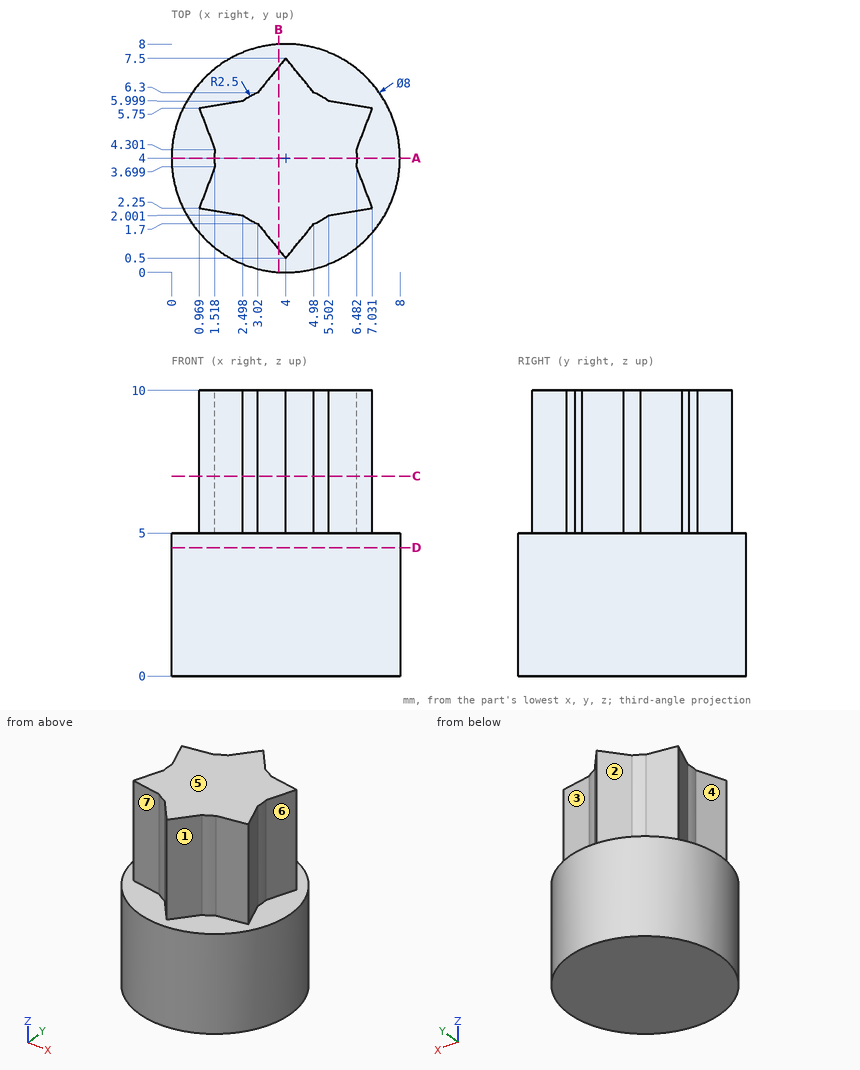
Verification items for this drawing (mm, ordinates from the low corner). A direction names the side the tool comes from. Coordinates: 2 decimals unless noted, no trailing zeros. Order: outer loops, then holes, each group sorted by start corner. A loop starts at its lowest first (then second) coordinate and runs counter-clockwise, first axis right, second up. Notation, with made-up numbers: (7.5, 23) - (59.5, 23) arc R8 cw to (59.5, 35) - close; hole circle Ø5 at (-19.75, 6.5). An arc over 180 degrees is marked (long way). Answer as a JSON object with one key per item and string values. Group by question number.
Item 1: Tool access check on the marked faces 1, 2 and 3. Record the directions out of +Z, -Z, +X, -X, +Y, -Y that give a thin tool (end or side, any length) a straight path to the whole face; none if there is none.
Item 2: Sectioned sample at C-C, the plane z = 7. Record the cut outline in (x, y), and give its area (3 significant figures).
Item 3: Depth check by flat-ended pin: pin 1 Ø3 at (y, z) = (6.5, 1) entering from -X; pin 2 Ø1.5 at (x, z) = (2.5, 6) entering from +Y; pin 3 Ø4 at (x, z) = (1, 2) entering from +Y. Enter the tip coordinate at first touch or a pass-through.
Item 4: Sectioned sample at A-A, the plane y = 4. Record the cut outline in (x, z).
Item 5: Draft check along Y on the marked faces 4, 5, 6 and 7. Enter one of: +Y half, -Y half, draft (parallel to the pull), parting line (faces both ways), or undercut.
Item 6: Scan lines: probe 1 along X at (y, z) = (4, 7.25); probe 2 along Z at (x, y) = (5.5, 6.25); probe 3 along Y at (x, z) = (2, 1.5) (1 decimal). Record each from-to range of solid material in increasing order.
Item 7: Sectioned sample at B-B, the plane x = 3.75. Record the cut outline in (y, z).
Item 8: Sectioned sample at D-D, the plane z = 4.5. Record the cut outline in (x, y).
Resolved:
{
 "1": {"face 1": "+Z, +X, -Y", "face 2": "+Z, -X, +Y", "face 3": "+Z, +X, +Y"},
 "2": {"outline": "(0.97, 2.25) - (2.5, 2) arc R2.5 ccw to (3.02, 1.7) - (4, 0.5) - (4.98, 1.7) arc R2.5 ccw to (5.5, 2) - (7.03, 2.25) - (6.48, 3.7) arc R2.5 ccw to (6.48, 4.3) - (7.03, 5.75) - (5.5, 6) arc R2.5 ccw to (4.98, 6.3) - (4, 7.5) - (3.02, 6.3) arc R2.5 ccw to (2.5, 6) - (0.97, 5.75) - (1.52, 4.3) arc R2.5 ccw to (1.52, 3.7) - close", "area": "25.1 mm^2"},
 "3": {"pin 1": "x = 0.13", "pin 2": "y = 6.58", "pin 3": "y = 7.87"},
 "4": {"outline": "(0, 0) - (8, 0) - (8, 5) - (6.5, 5) - (6.5, 10) - (1.5, 10) - (1.5, 5) - (0, 5) - close"},
 "5": {"face 4": "undercut", "face 5": "draft", "face 6": "undercut", "face 7": "-Y half"},
 "6": {"probe 1": "1.5 to 6.5", "probe 2": "0 to 5", "probe 3": "0.5 to 7.5"},
 "7": {"outline": "(0.01, 0) - (7.99, 0) - (7.99, 5) - (7.19, 5) - (7.19, 10) - (0.81, 10) - (0.81, 5) - (0.01, 5) - close"},
 "8": {"outline": "circle Ø8 at (4, 4)"}
}
